Model file for the job. Use its own axes, mm. Round coordinates to 2 decimals unless told otherwise and drop trailing zeros. Order: outer loops, then holes, each group sorted by start corner. A loop starts at its lowest first (then second) coordinate and runs counter-clockwise, first axis right, second up. Notation, with made-up numbers: M -38,-22.5 L 13,-22.5 A14 ccw 13,-3.5 Z; hole C 44.25,78 d10. An arc over 180 degrees is marked long. Return JSON: item names as keys, results as strings. Group by question number.
Item 1: Slice it at B-B on z = -63. Write the cut outline in (x, y).
Item 2: Slice it at A-A on x = -633.5. Write the cut outline in (y, z).
Item 3: Pin check, flat tips, straight feed: pin 1 Ø2 at (x, z) = (-673.5, -118) entering from -Y; pin 2 Ø4 at (x, z) = (-1242, -121.5) entering from +Y; pin 3 Ø5 at (x, y) = (-1151, 456) entering from +Z. Stop position of each tip, or through.
Item 4: Probe line 1 along Y through (x, z) = (-1639, -34); line 2 along Y through (x, z) = (-1636.5, 2); line 3 along Z through (x, y) = (-430, 492) (3 decimals). List the from-to ranges inside material, lowest first.
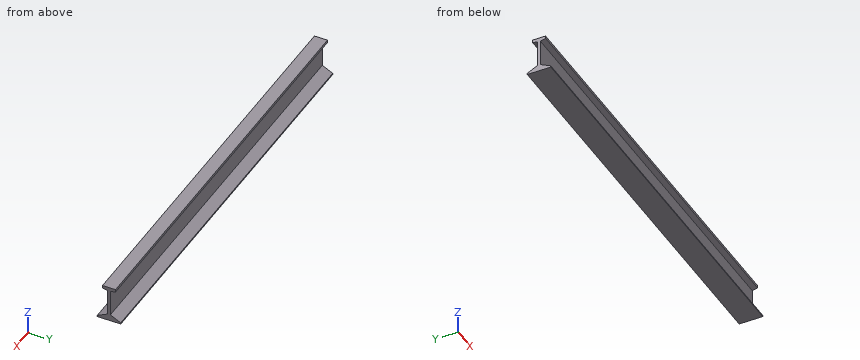
Autodesk Inventor part; units mm, degrees
ref_plane "YZ Plane" through (0, 0, 0) normal (1, 0, 0) x (0, 1, 0)
ref_plane "XZ Plane" through (0, 0, 0) normal (0, 1, 0) x (-1, 0, 0)
ref_plane "XY Plane" through (0, 0, 0) normal (0, 0, 1) x (1, 0, 0)
sketch "Sketch1" plane through (0, -4876.8, 165.1) normal (1, 0, 0) x (0, 1, 0)
  line L0 (0, 0) -> (0, -127)
  line L1 (9753.6, 0) -> (9753.6, -127)
  line L2 (9753.6, -152.4) -> (0, -152.4)
  line L3 (5410.2, -152.4) -> (5410.2, -165.1)
  line L4 (5410.2, -165.1) -> (5384.8, -171.45)
  line L5 (5384.8, -171.45) -> (5384.8, -298.45)
  line L6 (5384.8, -298.45) -> (5435.6, -323.85)
  line L7 (5435.6, -323.85) -> (5435.6, -330.2)
  line L8 (5435.6, -330.2) -> (5321.3, -330.2)
  line L9 (5321.3, -330.2) -> (5321.3, -323.85)
  line L10 (5372.1, -298.45) -> (5372.1, -171.45)
  line L11 (5410.2, -152.4) -> (5346.7, -152.4)
  line L12 (5378.45, -325.0091) -> (5378.45, -152.4) construction
  line L13 (5372.1, -171.45) -> (5346.7, -165.1)
  line L14 (5346.7, -165.1) -> (5346.7, -152.4)
  line L15 (5372.1, -298.45) -> (5384.8, -298.45) construction
  line L16 (5321.3, -323.85) -> (5372.1, -298.45)
  point P0 (9753.6, -50.8)
  point P1 (9753.6, -63.5)
  dimension "d8" = 12.7
  dimension "d6" = 6.35
  dimension "d17" = 6.35
  dimension "d12" = 6.35
  dimension "d14" = 50.8
  dimension "d13" = 25.4
  dimension "d16" = 25.4
  dimension "d5" = 25.4
  dimension "d11" = 6.35
  dimension "d10" = 50.8
  dimension "d3" = 90
  dimension "d15" = 127
  dimension "d7" = 177.8
  dimension "d9" = 127
  dimension "d4" = 6.35
  dimension "d2" = 4368.8
extrude "Extrusion1" add sketch "Sketch1" along normal blind 120.65 and the other way blind 1866.9
properties part number "Short I-Beam" material "Steel ASTM A36"
Output values:
{
 "1": {"outline": "M -1866.9,495.3 L 120.65,495.3 L 120.65,508 L -1866.9,508 Z"},
 "2": {"outline": "M 444.5,-165.1 L 558.8,-165.1 L 558.8,-158.75 L 508,-133.35 L 508,-6.35 L 533.4,0 L 533.4,12.7 L 469.9,12.7 L 469.9,0 L 495.3,-6.35 L 495.3,-133.35 L 444.5,-158.75 Z"},
 "3": {"pin 1": "y = 495.3", "pin 2": "y = 508", "pin 3": "z = -151.75"},
 "4": {"line 1": "495.3 to 508", "line 2": "469.9 to 533.4", "line 3": "-165.1 to -135, -5.525 to 12.7"}
}
